from build123d import *

# Parameters (mm, degrees)
SKETCH1_R               = 4.85
BOSS_EXTRUDE1_DEPTH     = 28
SKETCH2_W               = 2.36
SKETCH2_H               = 10
CUT_EXTRUDE1_DEPTH      = 14
CUT_EXTRUDE2_DEPTH      = 30.049671255
CUT_EXTRUDE2_DEPTH_BACK = 30.049671255
SKETCH3_R               = 1.575
BOSS_EXTRUDE2_DEPTH     = 3
SKETCH6_R               = 2.275
BOSS_EXTRUDE3_DEPTH     = 16
CUT_EXTRUDE3_START      = -6
SKETCH7_R               = 2.275
CUT_EXTRUDE3_DEPTH      = 6


with BuildPart() as part:
    # Sketch1 → Boss-Extrude1 (new body)
    with BuildSketch(Plane.XY):
        Circle(SKETCH1_R)
    extrude(amount=BOSS_EXTRUDE1_DEPTH)

    # Sketch2 → Cut-Extrude1 (cut)
    with BuildSketch(Plane.XY.offset(28)):
        Rectangle(SKETCH2_W, SKETCH2_H)
    extrude(amount=-CUT_EXTRUDE1_DEPTH, mode=Mode.SUBTRACT)

    # Sketch3 → Cut-Extrude2 (cut, two sides: drawn at the far end of the back side and taken through both)
    with BuildSketch(Plane.ZY.offset(-1.18).offset(-CUT_EXTRUDE2_DEPTH_BACK)):
        with Locations((23, 0)):
            Circle(SKETCH3_R)
    extrude(amount=CUT_EXTRUDE2_DEPTH + CUT_EXTRUDE2_DEPTH_BACK, mode=Mode.SUBTRACT)

    # Sketch5 → Boss-Extrude2 (add)
    with BuildSketch(Plane(origin=(0, 0, 0), x_dir=(-1, 0, 0), z_dir=(0, 0, -1))):
        Polygon((-2.309401077, -4), (-14, -4), (-14, 4), (-2.309401077, 4), (3.535898385, 14.124355653), (10.464101615, 10.124355653), (4.618802154, 0), (10.464101615, -10.124355653), (3.535898385, -14.124355653), align=None)
    extrude(amount=BOSS_EXTRUDE2_DEPTH)

    # Sketch6 → Boss-Extrude3 (add)
    with BuildSketch(Plane.XY):
        with Locations((-5, 8.660254038)):
            Circle(SKETCH6_R)
        with Locations((-5, -8.660254038)):
            Circle(SKETCH6_R)
        with Locations((10, 0)):
            Circle(SKETCH6_R)
    extrude(amount=BOSS_EXTRUDE3_DEPTH)

    # Sketch7 → Cut-Extrude3 (cut)
    with BuildSketch(Plane.XY.offset(16).offset(CUT_EXTRUDE3_START)):
        with Locations((-5, 8.660254038)):
            Circle(SKETCH7_R)
    extrude(amount=CUT_EXTRUDE3_DEPTH, mode=Mode.SUBTRACT)


solid = part.part
Geometry: final body of the model. Coordinates: model frame, mm. A direction names the side the tool comes from. Give positions to 0.01 mm unless a question says otherwise; leave off trailing zeros. Write each loop counter-clockwise with the first axis right and the second up, starting at its lowest first coordinate (ties: lowest second). Pieces come first, ordered by that corner, then holes. Notation, with made-up numbers: (-23.75, 3) -> (-7.75, 3) arc R17 cw to (-7.75, 30) -> close; hole circle Ø8 at (3, 60.25). An arc over 180 degrees is marked (long way). Answer as a JSON object with one key per item and string values.
1. Cut plane C-C on y = 1. Output: boundary loops of the cut face in (x, z).
Ans:
{"outline": "(-5.2, -3) -> (14, -3) -> (14, 0) -> (12.04, 0) -> (12.04, 16) -> (7.96, 16) -> (7.96, 0) -> (4.75, 0) -> (4.75, 21.78) -> (1.18, 21.78) -> (1.18, 14) -> (-1.18, 14) -> (-1.18, 21.78) -> (-4.75, 21.78) -> (-4.75, 0) -> (-5.2, 0) -> close; (-4.75, 24.22) -> (-1.18, 24.22) -> (-1.18, 28) -> (-4.75, 28) -> close; (1.18, 24.22) -> (4.75, 24.22) -> (4.75, 28) -> (1.18, 28) -> close"}
2. Cut plane D-D on y = -3.25. Output: boundary loops of the cut face in (x, z), and give its area (3 significant figures).
Ans:
{"outline": "(-6.5, -3) -> (14, -3) -> (14, 0) -> (3.6, 0) -> (3.6, 28) -> (1.18, 28) -> (1.18, 14) -> (-1.18, 14) -> (-1.18, 28) -> (-3.6, 28) -> (-3.6, 0) -> (-6.5, 0) -> close", "area": "230 mm^2"}
3. Ray query, probe 1 along Z at (x, y) = (-2.9, 0) (3 decimals); probe 2 along Y at (x, z) = (2.1, 23) (3 decimals); probe 3 along Z at (x, y) = (-5, -8.25). Return the intervals inside material, ascending. Write a range as from..to.
Ans:
{"probe 1": "z = -3..21.425, 24.575..28", "probe 2": "y = -4.372..-1.575, 1.575..4.372", "probe 3": "z = -3..16"}
4. Access query for faces 1 (the flat face through (-5, 9, 10)), 2 (the flat face through (0, 0, 14)), 3 (the flat face through (-5, -9, 16)), 4 (the flat face through (-4, 6, 0)). Directions: +Z, -Z, +X, -X, +Y, -Y. A direction counts if a zero-diameter tool reaches every point of the face in a straight line with its end or side. Return the directions, or none.
Ans:
{"face 1": "+Z, +X, -X, +Y", "face 2": "+Z, +Y, -Y", "face 3": "+Z, +X, -X, -Y", "face 4": "+Z"}
5. Mould query, pull axis Y, two halves, no side actions, for faces 5 (the flat face through (-6.952, 12.152, -1.479)), 6 (the flat face through (10, 0, 16)), 7 (the cylindrical face through (-5.49, -10.88, 7.89)). Classes: pulls with the +Y half, pulls with the -Y half, needs draft (parallel to the pull), parting line crosses it, or undercut.
Ans:
{"face 5": "pulls with the +Y half", "face 6": "needs draft", "face 7": "undercut"}
6. Cut plane B-B on z = 23. Output: boundary loops of the cut face in (x, y) (3 decimals).
Ans:
{"outline": "(-4.587, -1.575) arc R4.85 ccw to (-1.18, -4.704) -> (-1.18, -1.575) -> close; (-4.587, 1.575) -> (-1.18, 1.575) -> (-1.18, 4.704) arc R4.85 ccw to start; (1.18, -4.704) arc R4.85 ccw to (4.587, -1.575) -> (1.18, -1.575) -> close; (1.18, 1.575) -> (4.587, 1.575) arc R4.85 ccw to (1.18, 4.704) -> close"}
7. Contact query for flat-ended pins moving along their axis: pin 1 (4 mm diameter, centred on y = 0, z = 23, fed in from +X); pin 2 (7.5 mm diameter, centred on y = -1.5, z = 18, fed in from -X); pin 3 (6.5 mm diameter, centred on x = -5.5, y = 8.5, fed in from +Z); pin 4 (8 mm diameter, centred on x = 7.5, y = 10, fed in from +Z). Output: stop coordinate, or through.
Ans:
{"pin 1": "stops at x = 4.85", "pin 2": "stops at x = -4.85", "pin 3": "stops at z = 10", "pin 4": "passes through"}
8. Cut plane A-A on x = 0. Output: boundary loops of the cut face in (y, z), and give its area (3 significant figures).
Ans:
{"outline": "(-8, -3) -> (8, -3) -> (8, 0) -> (4.85, 0) -> (4.85, 14) -> (-4.85, 14) -> (-4.85, 0) -> (-8, 0) -> close", "area": "184 mm^2"}
